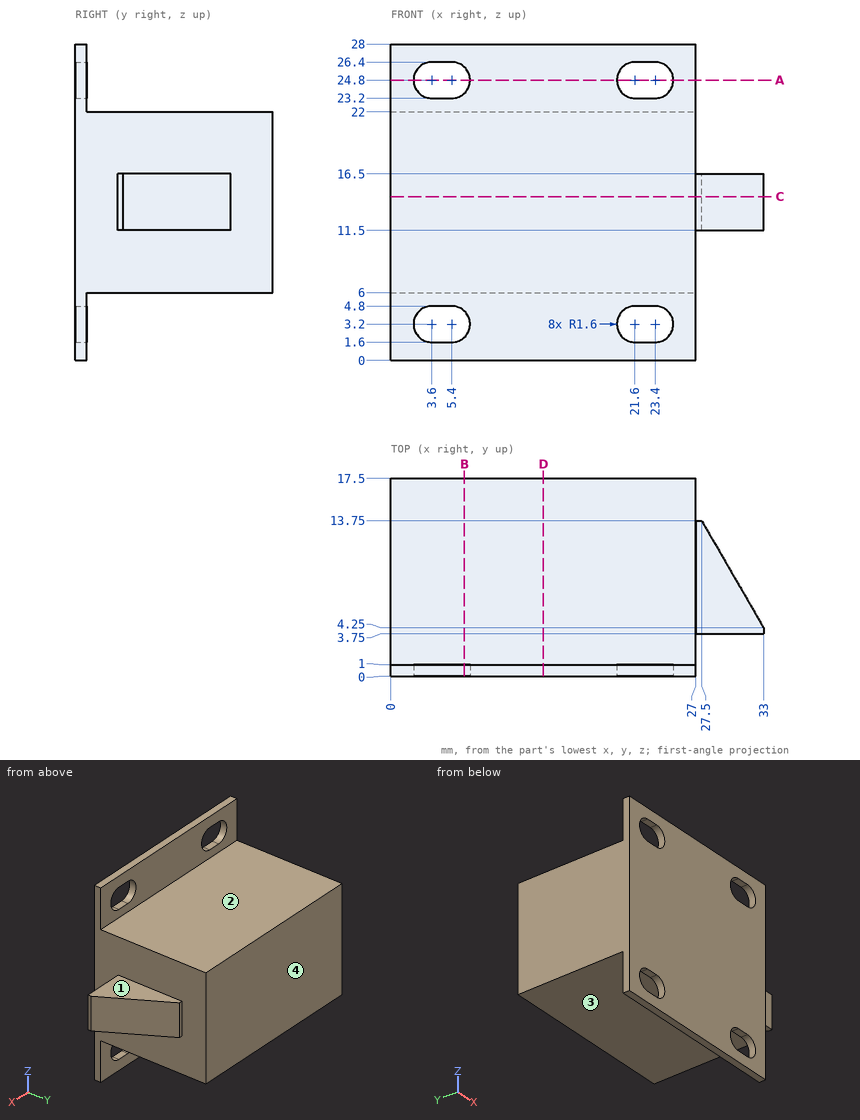
Design review of the part shown in the three views and the two pictorial views. Dimensions are in mm from the part's minimum x, y and z. A direction names the side the tool comes from. Round coordinates to 2 decimals unless told otherwise and drop trailing zeros. Loops run counter-clockwise (first coordinate to the right, second up) from the corner with the lowest first, then second, coordinate; pieces in that order, holes last. Notation, with made-up numbers: (63.5, 24.25) - (94.5, 24.25) arc R14 ccw to (94.5, 34.25) - close; hole circle Ø7 at (-39.75, 57.5). An arc over 180 degrees is marked (long way). One line per item, written item: value. Start each with the question number.
Item 1: Take a section at A-A (z = 24.8). Give the boundary of the cut face in (x, y), plus the area to 3 significant figures.
Item 2: Clearance check with flat-ended pins moving along their axes: pin 1 Ø8 at (x, y) = (7, 7.5) entering from -Z; pin 2 Ø5 at (x, y) = (14, 6.5) entering from +Z; pin 3 Ø1.5 at (x, z) = (28.5, 14.5) entering from -Y. State where each tip first meets the part, or that it passes through.
Item 3: Take a section at C-C (z = 14.5). Give the boundary of the cut face in (x, y), plus the area to 3 significant figures.
Item 4: Take a section at D-D (x = 13.5). Give the boundary of the cut face in (y, z), plus the area to 3 significant figures.
Item 5: For the marked faces 1, 2, 3 and 4, list the 3-axis set-ups (+Z, -Z, +X, -X, +Y, -Y) from which the entire face can be reached by the end or side of a thin tool; tool diameter is ignored.
Item 6: For L1, parallel to Z at x = 3.5, y = 3.25; L2, parallel to X at y = 14, z = 8.75; L3, parallel to Y at x = 24, z = 22.75, list the stretches that pass through material, from the lowest coordinate up.
Item 7: Take a section at B-B (x = 6.5). Give the boundary of the cut face in (y, z), plus the area to 3 significant figures.
Answer below:
1. outline: (0, 0) - (2, 0) - (2, 1) - (0, 1) - close; (7, 0) - (20, 0) - (20, 1) - (7, 1) - close; (25, 0) - (27, 0) - (27, 1) - (25, 1) - close
1. area: 17.0 mm2
2. pin 1: stops at z = 6
2. pin 2: stops at z = 22
2. pin 3: stops at y = 3.75
3. outline: (0, 0) - (27, 0) - (27, 3.75) - (33, 3.75) - (33, 4.25) - (27.5, 13.75) - (27, 13.75) - (27, 17.5) - (0, 17.5) - close
3. area: 506 mm2
4. outline: (0, 0) - (1, 0) - (1, 6) - (17.5, 6) - (17.5, 22) - (1, 22) - (1, 28) - (0, 28) - close
4. area: 292 mm2
5. face 1: +Z, +X, +Y, -Y
5. face 2: +Z, +X, -X, +Y
5. face 3: -Z, +X, -X, +Y
5. face 4: +Z, -Z, +X, -X, +Y
6. L1: z = 6 to 22
6. L2: x = 0 to 27
6. L3: y = 0 to 1
7. outline: (0, 0) - (1, 0) - (1, 2.04) - (0, 2.04) - close; (0, 4.36) - (1, 4.36) - (1, 6) - (17.5, 6) - (17.5, 22) - (1, 22) - (1, 23.64) - (0, 23.64) - close; (0, 25.96) - (1, 25.96) - (1, 28) - (0, 28) - close
7. area: 287 mm2
